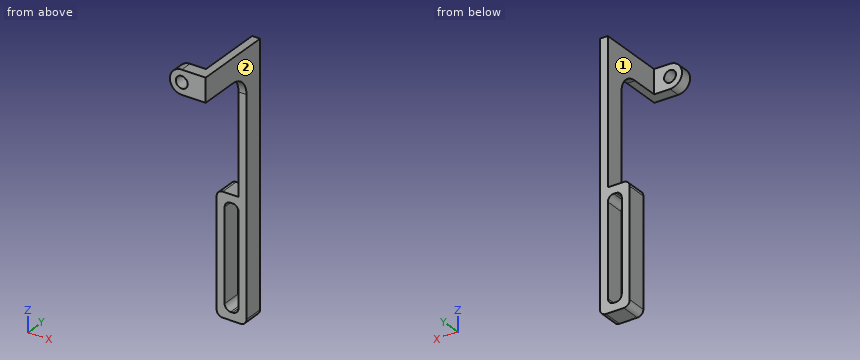
from build123d import *

# Parameters (mm, degrees)
SKETCH_1_R      = 3
SKETCH_1_R_2    = 1.5
EXTRUDE_1_DEPTH = 3
SKETCH_2_W      = 2
SKETCH_2_H      = 6
EXTRUDE_2_DEPTH = 15
SKETCH_3_W      = 3.5
SKETCH_3_H      = 26
EXTRUDE_3_DEPTH = 5
FILLET_1_R      = 5
FILLET_2_R      = 1.5
FILLET_3_R      = 1.5


with BuildPart() as part:
    # 草图1 → 凸台-拉伸1 (new body)
    # profile 1 of 2: a face of its own
    with BuildSketch(Plane(origin=(0, 0, 0), x_dir=(1, 0, 0), z_dir=(0, 1, 0))):
        Circle(SKETCH_1_R)
        with Locations(Location((0, 0, 0), (0, 0, 270))):
            Circle(SKETCH_1_R_2, mode=Mode.SUBTRACT)
    # profile 2 of 2: a face of its own
    with BuildSketch(Plane(origin=(0, 0, 0), x_dir=(1, 0, 0), z_dir=(0, 1, 0))):
        with BuildLine():
            Line((6, 3), (0, 3))
            ThreePointArc((0, 3), (2.121320344, 2.121320344), (3, 0))
            ThreePointArc((3, 0), (2.121320344, -2.121320344), (0, -3))
            Line((0, -3), (6, -3))
            Line((6, -3), (6, 3))
        make_face()
    extrude(amount=EXTRUDE_1_DEPTH)

    # 草图2 → 凸台-拉伸2 (add)
    with BuildSketch(Plane(origin=(0, 0, 0), x_dir=(1, 0, 0), z_dir=(0, 1, 0))):
        with Locations((5, 0)):
            Rectangle(SKETCH_2_W, SKETCH_2_H)
    extrude(amount=EXTRUDE_2_DEPTH)

    # 草图3 → 凸台-拉伸3 (add)
    with BuildSketch(Plane(origin=(0, 15, 0), x_dir=(1, 0, 0), z_dir=(0, 1, 0))):
        Polygon((6, -3), (6, 63), (4, 63), (-1.5, 63), (-1.5, 33), (4, 33), (4, -3), align=None)
        with Locations((2.25, 48)):
            Rectangle(SKETCH_3_W, SKETCH_3_H, mode=Mode.SUBTRACT)
    extrude(amount=EXTRUDE_3_DEPTH)

    # 圆角1
    fillet_1_edges = [part.edges().sort_by_distance(p)[0] for p in [
        (5, 15, -3),
    ]]
    fillet(fillet_1_edges, radius=FILLET_1_R)

    # 圆角2
    fillet_2_edges = [part.edges().sort_by_distance(p)[0] for p in [
        (6, 17.5, -63),
        (-1.5, 17.5, -63),
        (-1.5, 17.5, -33),
        (0.5, 17.5, -35),
        (4, 17.5, -35),
    ]]
    fillet(fillet_2_edges, radius=FILLET_2_R)

    # 圆角3
    fillet_3_edges = [part.edges().sort_by_distance(p)[0] for p in [
        (4, 17.5, -61),
        (0.5, 17.5, -61),
    ]]
    fillet(fillet_3_edges, radius=FILLET_3_R)


solid = part.part
Can you work these out from the model? Positions are in its coordinate system, mm. Face numbers are marked on the shaded views. A direction names the side the tool comes from. Coordinates: 2 decimals unless noted, no trailing zeros. Write each loop counter-clockwise with the first axis right and the second up, starting at its lowest first coordinate (ties: lowest second). Pieces come first, ordered by that corner, then holes. Notation, with made-up numbers: (26, -25) -> (59, -25) arc R22 ccw to (59, -1) -> close; hole circle Ø2 at (59.5, 39). An arc over 180 degrees is marked (long way). Answer as CSV lines item,"result".
1) If we section it at D-D on z = -58: Please give me the cut outline in (x, y).
Check result:
outline,"(-1.5, 15) -> (0.5, 15) -> (0.5, 20) -> (-1.5, 20) -> close; (4, 15) -> (6, 15) -> (6, 20) -> (4, 20) -> close"
2) If we section it at C-C on x = -0.75: Please give me the cut outline in (y, z).
Check result:
outline,"(0, -2.9) -> (3, -2.9) -> (3, -1.3) -> (0, -1.3) -> close; (0, 1.3) -> (3, 1.3) -> (3, 2.9) -> (0, 2.9) -> close; (15, -62.8) -> (20, -62.8) -> (20, -33.2) -> (15, -33.2) -> close"
3) Will these pins go through, and if not, where does the flat tip stop? P1, Ø5, axis at y = 11.5, z = -20, coming from the -X side; P2, Ø3, axis at x = 3, y = 3.5, coming from the -Z side; P3, Ø1.5, axis at x = 4.5, z = -12, coming from the -Y side; P4, Ø4, axis at y = 18, z = -46.5, coming from the -X side.
Check result:
P1,"through"
P2,"z = -3"
P3,"y = 15"
P4,"x = -1.5"
4) On a 3-axis mill with a long thin cutter (end or side, diameter ignored), from which of +Z, -Z, +X, -X, +Y, -Y can I reach the whole of each face in a straight line? I mean the marked faces 1 and 2. Say none if no direction works.
Check result:
face 1,"+Z, -X, +Y"
face 2,"+Z, -Z, +X, +Y, -Y"
5) If I drill on line 1 (X direction, y = 0.9, z = 0); line 2 (X direction, y = 16.25, z = -40); line 3 (Y direction, x = 1.5, z = -35), over which ranges is the centre line in solid material (lowest first)? Write a range as from..to.
Check result:
line 1,"-3..-1.5, 1.5..6"
line 2,"-1.5..0.5, 4..6"
line 3,"15..20"
6) If we section it at A-A on z = 0: Please give me the cut outline in (x, y), then the cut area to 3 significant figures.
Check result:
outline,"(-3, 0) -> (-1.5, 0) -> (-1.5, 3) -> (-3, 3) -> close; (1.5, 0) -> (6, 0) -> (6, 20) -> (4, 20) -> (4, 3) -> (1.5, 3) -> close"
area,"52.0 mm²"
7) If we section it at B-B on y = 18.25: Please give me the cut outline in (x, z), then the cut area to 3 significant figures.
Check result:
outline,"(-1.5, -61.5) arc R1.5 ccw to (0, -63) -> (4.5, -63) arc R1.5 ccw to (6, -61.5) -> (6, 3) -> (4, 3) -> (4, -33) -> (0, -33) arc R1.5 ccw to (-1.5, -34.5) -> close; hole (0.5, -59.5) arc R1.5 ccw to (2, -61) -> (2.5, -61) arc R1.5 ccw to (4, -59.5) -> (4, -36.5) arc R1.5 ccw to (2.5, -35) -> (2, -35) arc R1.5 ccw to (0.5, -36.5) -> close"
area,"206 mm²"
